from build123d import *

# Parameters (mm, degrees)
SKETCH_1_W          = 72
SKETCH_1_H          = 100
EXTRUDE_1_DEPTH     = 8
CUT_EXTRUDE_1_REACH = 64.129
SKETCH_2_R          = 2.2
SKETCH_2_W          = 56
SKETCH_2_H          = 26
EXTRUDE_2_DEPTH     = 8
SKETCH_4_W          = 72
SKETCH_4_H          = 84
EXTRUDE_3_DEPTH     = 8
SKETCH_5_R          = 2.2
SKETCH_5_W          = 56
SKETCH_5_H          = 26
CUT_EXTRUDE_2_DEPTH = 8
EXTRUDE_4_DEPTH     = 8


with BuildPart() as part:
    # 草图1 → 凸台-拉伸1 (new body)
    with BuildSketch(Plane.XY):
        Rectangle(SKETCH_1_W, SKETCH_1_H)
    extrude(amount=EXTRUDE_1_DEPTH)

    # 草图2 → 切除-拉伸1 (cut, up to next)
    with BuildSketch(Plane.XY.offset(8), mode=Mode.PRIVATE) as cut_extrude_1_sk1:
        with Locations((-26, -42)):
            Circle(SKETCH_2_R)
    cut_extrude_1_tool1 = extrude(cut_extrude_1_sk1.sketch, amount=-CUT_EXTRUDE_1_REACH, mode=Mode.PRIVATE) & part.part
    # 草图2 → 切除-拉伸1 (cut, up to next)
    with BuildSketch(Plane.XY.offset(8), mode=Mode.PRIVATE) as cut_extrude_1_sk2:
        with Locations((0, -42)):
            Circle(SKETCH_2_R)
    cut_extrude_1_tool2 = extrude(cut_extrude_1_sk2.sketch, amount=-CUT_EXTRUDE_1_REACH, mode=Mode.PRIVATE) & part.part
    # 草图2 → 切除-拉伸1 (cut, up to next)
    with BuildSketch(Plane.XY.offset(8), mode=Mode.PRIVATE) as cut_extrude_1_sk3:
        with Locations((26, -42)):
            Circle(SKETCH_2_R)
    cut_extrude_1_tool3 = extrude(cut_extrude_1_sk3.sketch, amount=-CUT_EXTRUDE_1_REACH, mode=Mode.PRIVATE) & part.part
    # 草图2 → 切除-拉伸1 (cut, up to next)
    with BuildSketch(Plane.XY.offset(8), mode=Mode.PRIVATE) as cut_extrude_1_sk4:
        with Locations((26, 42)):
            Circle(SKETCH_2_R)
    cut_extrude_1_tool4 = extrude(cut_extrude_1_sk4.sketch, amount=-CUT_EXTRUDE_1_REACH, mode=Mode.PRIVATE) & part.part
    # 草图2 → 切除-拉伸1 (cut, up to next)
    with BuildSketch(Plane.XY.offset(8), mode=Mode.PRIVATE) as cut_extrude_1_sk5:
        with Locations((0, 42)):
            Circle(SKETCH_2_R)
    cut_extrude_1_tool5 = extrude(cut_extrude_1_sk5.sketch, amount=-CUT_EXTRUDE_1_REACH, mode=Mode.PRIVATE) & part.part
    # 草图2 → 切除-拉伸1 (cut, up to next)
    with BuildSketch(Plane.XY.offset(8), mode=Mode.PRIVATE) as cut_extrude_1_sk6:
        with Locations((-26, 42)):
            Circle(SKETCH_2_R)
    cut_extrude_1_tool6 = extrude(cut_extrude_1_sk6.sketch, amount=-CUT_EXTRUDE_1_REACH, mode=Mode.PRIVATE) & part.part
    # 草图2 → 切除-拉伸1 (cut, up to next)
    with BuildSketch(Plane.XY.offset(8), mode=Mode.PRIVATE) as cut_extrude_1_sk7:
        with Locations((-26, 0)):
            Circle(SKETCH_2_R)
    cut_extrude_1_tool7 = extrude(cut_extrude_1_sk7.sketch, amount=-CUT_EXTRUDE_1_REACH, mode=Mode.PRIVATE) & part.part
    # 草图2 → 切除-拉伸1 (cut, up to next)
    with BuildSketch(Plane.XY.offset(8), mode=Mode.PRIVATE) as cut_extrude_1_sk8:
        Circle(SKETCH_2_R)
    cut_extrude_1_tool8 = extrude(cut_extrude_1_sk8.sketch, amount=-CUT_EXTRUDE_1_REACH, mode=Mode.PRIVATE) & part.part
    # 草图2 → 切除-拉伸1 (cut, up to next)
    with BuildSketch(Plane.XY.offset(8), mode=Mode.PRIVATE) as cut_extrude_1_sk9:
        with Locations((26, 0)):
            Circle(SKETCH_2_R)
    cut_extrude_1_tool9 = extrude(cut_extrude_1_sk9.sketch, amount=-CUT_EXTRUDE_1_REACH, mode=Mode.PRIVATE) & part.part
    # 草图2 → 切除-拉伸1 (cut, up to next)
    with BuildSketch(Plane.XY.offset(8), mode=Mode.PRIVATE) as cut_extrude_1_sk10:
        with Locations((0, 21)):
            Rectangle(SKETCH_2_W, SKETCH_2_H)
    cut_extrude_1_tool10 = extrude(cut_extrude_1_sk10.sketch, amount=-CUT_EXTRUDE_1_REACH, mode=Mode.PRIVATE) & part.part
    # 草图2 → 切除-拉伸1 (cut, up to next)
    with BuildSketch(Plane.XY.offset(8), mode=Mode.PRIVATE) as cut_extrude_1_sk11:
        with Locations((0, -21)):
            Rectangle(SKETCH_2_W, SKETCH_2_H)
    cut_extrude_1_tool11 = extrude(cut_extrude_1_sk11.sketch, amount=-CUT_EXTRUDE_1_REACH, mode=Mode.PRIVATE) & part.part
    add(cut_extrude_1_tool1.solids().sort_by_distance((-26, -42, 8))[0], mode=Mode.SUBTRACT)
    add(cut_extrude_1_tool2.solids().sort_by_distance((0, -42, 8))[0], mode=Mode.SUBTRACT)
    add(cut_extrude_1_tool3.solids().sort_by_distance((26, -42, 8))[0], mode=Mode.SUBTRACT)
    add(cut_extrude_1_tool4.solids().sort_by_distance((26, 42, 8))[0], mode=Mode.SUBTRACT)
    add(cut_extrude_1_tool5.solids().sort_by_distance((0, 42, 8))[0], mode=Mode.SUBTRACT)
    add(cut_extrude_1_tool6.solids().sort_by_distance((-26, 42, 8))[0], mode=Mode.SUBTRACT)
    add(cut_extrude_1_tool7.solids().sort_by_distance((-26, 0, 8))[0], mode=Mode.SUBTRACT)
    add(cut_extrude_1_tool8.solids().sort_by_distance((0, 0, 8))[0], mode=Mode.SUBTRACT)
    add(cut_extrude_1_tool9.solids().sort_by_distance((26, 0, 8))[0], mode=Mode.SUBTRACT)
    add(cut_extrude_1_tool10.solids().sort_by_distance((0, 21, 8))[0], mode=Mode.SUBTRACT)
    add(cut_extrude_1_tool11.solids().sort_by_distance((0, -21, 8))[0], mode=Mode.SUBTRACT)

    # 草图3 → 凸台-拉伸2 (add)
    with BuildSketch(Plane.XY.offset(8)):
        Polygon((-28, 30.60122868), (-6.768682564, 21.407188314), (-28, 12.93157869), (-28, 8), (-24.288219299, 8), (-0.025829724, 18.487253581), (24.191837476, 8), (28, 8), (28, 11.903155093), (6.450556004, 21.286627452), (28, 30.60122868), (28, 34), (24.776184912, 34), (-0.016552798, 24.102660047), (-22.746110137, 34), (-28, 34), align=None)
        Polygon((-28, -8), (-24.288219299, -8), (-0.025829724, -18.487253581), (24.191837476, -8), (28, -8), (28, -11.903155093), (6.450556004, -21.286627452), (28, -30.60122868), (28, -34), (24.776184912, -34), (-0.016552798, -24.102660047), (-22.746110137, -34), (-28, -34), (-28, -30.60122868), (-6.768682564, -21.407188314), (-28, -12.93157869), align=None)
    extrude(amount=-EXTRUDE_2_DEPTH)

    # 草图4 → 凸台-拉伸3 (add)
    with BuildSketch(Plane.XY.offset(8)):
        with Locations((0, 92)):
            Rectangle(SKETCH_4_W, SKETCH_4_H)
    extrude(amount=-EXTRUDE_3_DEPTH)

    # 草图5 → 切除-拉伸2 (cut)
    with BuildSketch(Plane.XY.offset(8)):
        with Locations((0, 84)):
            Circle(SKETCH_5_R)
        with Locations((0, 126)):
            Circle(SKETCH_5_R)
        with Locations((26, 126)):
            Circle(SKETCH_5_R)
        with Locations((-26, 126)):
            Circle(SKETCH_5_R)
        with Locations((-26, 84)):
            Circle(SKETCH_5_R)
        with Locations((26, 84)):
            Circle(SKETCH_5_R)
        with Locations((0, 105)):
            Rectangle(SKETCH_5_W, SKETCH_5_H)
        with Locations((0, 63)):
            Rectangle(SKETCH_5_W, SKETCH_5_H)
    extrude(amount=-CUT_EXTRUDE_2_DEPTH, mode=Mode.SUBTRACT)

    # 草图6 → 凸台-拉伸4 (add)
    with BuildSketch(Plane.XY.offset(8)):
        Polygon((-23.974932243, 118), (0.019492881, 108.0358887), (23.327208426, 118), (28, 118), (28, 113.17961686), (8.109494179, 104.676371941), (28, 96.416486039), (28, 92), (22.06939562, 92), (-0.053196802, 101.186799516), (-21.542650648, 92), (-28, 92), (-28, 96.057479873), (-8.1431981, 104.546316276), (-28, 112.792206026), (-28, 118), align=None)
        Polygon((-23.547674388, 76), (0.012222409, 66.314841093), (22.812282036, 76), (28, 76), (28, 71.451887213), (8.089746155, 62.994278964), (28, 54.80943953), (28, 50), (23.327208426, 50), (0.037852996, 59.573942964), (-22.500390573, 50), (-28, 50), (-28, 54.415625486), (-8.03967075, 62.894505093), (-28, 71.099929858), (-28, 76), align=None)
    extrude(amount=-EXTRUDE_4_DEPTH)


solid = part.part
Design review of the part built by this model. Coordinates are the model's own, in mm. A direction names the side the tool comes from. Round coordinates to 2 decimals unless told otherwise and drop trailing zeros. Write each loop counter-clockwise with the first axis right and the second up, starting at its lowest first coordinate (ties: lowest second). Pieces come first, ordered by that corner, then holes. Notation, with made-up numbers: (-12.75, -24) - (10.25, -24) arc R11 ccw to (10.25, -15) - close; hole circle Ø4 at (-12.75, 11.5). An arc over 180 degrees is marked (long way). Use a Markdown table: item, result. Add a question column.
1. For faces 5 (the face through (18.194, 108.988, 4.056)), 6 (the face through (-7, 43, 8)), list the 3-axis set-ups (+Z, -Z, +X, -X, +Y, -Y) from which the entire face can be reached by the end or side of a thin tool; tool diameter is ignored.
2. Mouldability with a two-part tool opening along Y and no side actions: class faces 1 (the face through (-1, 134, 4)), 2 (the face through (-26.29, 86.18, 4.06)), 3 (the face through (17.376, -16.529, 4.056)), 4 (the face through (-36, 41, 4)) as +Y half, -Y half, draft (parallel to the pull), parting line (faces both ways), or undercut.
3. We need section B-B (z = 6). Count the separate pieces of the cut face and the enclosed holes in it, then the cut area to 3 significant figures.
4. Wall thickness on probe 1 along X at (y, z) = (55, 2.5); probe 2 along X at (y, z) = (41, 7); probe 3 along X at (y, z) = (23, 7): over which ranges is each line inside the solid? List them lowest first.
5. We need section C-C (y = 16). State the section outline as (x, z) points.
6. We need section A-A (y = 42). State the section outline as (x, z) points, then the cut area to 3 significant figures.
Output:
| question | item | result |
|---|---|---|
| 1 | face 5 | +Z, -Z |
| 1 | face 6 | +Z, +X, -X, +Y, -Y |
| 2 | face 1 | +Y half |
| 2 | face 2 | undercut |
| 2 | face 3 | undercut |
| 2 | face 4 | draft |
| 3 | separate pieces | 1 |
| 3 | enclosed holes | 31 |
| 3 | area | 9,720 mm2 |
| 4 | probe 1 | x = -36 to -28, -26.62 to -10.73, 11.16 to 27.54, 28 to 36 |
| 4 | probe 2 | x = -36 to -27.96, -24.04 to -1.96, 1.96 to 24.04, 27.96 to 36 |
| 4 | probe 3 | x = -36 to -28, -10.45 to 10.41, 28 to 36 |
| 5 | outline | (-36, 0) - (-28, 0) - (-28, 8) - (-36, 8) - close; (-20.31, 0) - (-5.78, 0) - (-5.78, 8) - (-20.31, 8) - close; (5.72, 0) - (18.59, 0) - (18.59, 8) - (5.72, 8) - close; (28, 0) - (36, 0) - (36, 8) - (28, 8) - close |
| 6 | outline | (-36, 0) - (-28.2, 0) - (-28.2, 8) - (-36, 8) - close; (-23.8, 0) - (-2.2, 0) - (-2.2, 8) - (-23.8, 8) - close; (2.2, 0) - (23.8, 0) - (23.8, 8) - (2.2, 8) - close; (28.2, 0) - (36, 0) - (36, 8) - (28.2, 8) - close |
| 6 | area | 470 mm2 |
